Part model, mm, in its own coordinate system. A direction names the side the tool comes from. Round coordinates to 2 decimals unless told otherwise and drop trailing zeros. Order: outer loops, then holes, each group sorted by start corner. A loop starts at its lowest first (then second) coordinate and runs counter-clockwise, first axis right, second up. Notation, with made-up numbers: (-22, 22.5) -> (10, 22.5) arc R15 ccw to (10, 47.5) -> close; hole circle Ø3 at (75, 70). An arc over 180 degrees is marked (long way). Return JSON: item names as keys, results as strings. Group by question number.
from build123d import *

# Parameters (mm, degrees)
SKETCH1_R           = 114.3
BOSS_EXTRUDE1_DEPTH = 76.2
SKETCH2_R           = 88.9
BOSS_EXTRUDE2_DEPTH = 25.4
SKETCH3_W           = 67.503621206
SKETCH3_H           = 186.628871474
BOSS_EXTRUDE3_DEPTH = 203.2
SKETCH4_R           = 76.2
CUT_EXTRUDE1_DEPTH  = 127
FILLET1_SIZE        = 25.4
FILLET2_SIZE        = 12.7


with BuildPart() as part:
    # Sketch1 → Boss-Extrude1 (new body)
    with BuildSketch(Plane(origin=(0, 0, 0), x_dir=(1, 0, 0), z_dir=(0, 1, 0))):
        with Locations(Location((0, 0, 0), (0, 0, 90))):
            Circle(SKETCH1_R)
    extrude(amount=BOSS_EXTRUDE1_DEPTH)

    # Sketch2 → Boss-Extrude2 (add)
    with BuildSketch(Plane(origin=(0, 0, 0), x_dir=(-1, 0, 0), z_dir=(0, -1, 0))):
        with Locations(Location((0, 0, 0), (0, 0, 90))):
            Circle(SKETCH2_R)
    extrude(amount=BOSS_EXTRUDE2_DEPTH)

    # Sketch3 → Boss-Extrude3 (add)
    with BuildSketch(Plane(origin=(0, 76.2, 0), x_dir=(1, 0, 0), z_dir=(0, 1, 0))):
        Rectangle(SKETCH3_W, SKETCH3_H)
    extrude(amount=BOSS_EXTRUDE3_DEPTH)

    # Sketch4 → Cut-Extrude1 (cut)
    with BuildSketch(Plane.ZY.offset(33.751810603)):
        with Locations((0, 177.8)):
            Circle(SKETCH4_R)
    extrude(amount=-CUT_EXTRUDE1_DEPTH, mode=Mode.SUBTRACT)

    # Fillet1
    # a fillet whose section is not a circle: 25.4 mm, written as the material it takes off along each edge
    with BuildSketch(Plane(origin=(97.251810603, 279.4, 93.314435737), x_dir=(0, -1, 0), z_dir=(-1, 0, 0)), Plane(origin=(-97.251810603, 279.4, -93.314435737), x_dir=(0, -1, 0), z_dir=(1, 0, 0))) as fillet1_piece_1:
        with BuildLine():
            Bezier((FILLET1_SIZE, 0), (0, 0), (0, -FILLET1_SIZE), weights=[1, 1, 1])
            Line((0, -FILLET1_SIZE), (0, 0))
            Line((0, 0), (FILLET1_SIZE, 0))
        make_face()
    extrude(amount=194.503621206, mode=Mode.SUBTRACT)

    # Fillet2
    # a fillet whose section is not a circle: 12.7 mm, written as the material it adds along each edge
    with BuildSketch(Plane(origin=(33.751810603, 76.2, 93.314435737), x_dir=(0, 0, 1), z_dir=(-1, 0, 0)), Plane(origin=(-33.751810603, 76.2, -93.314435737), x_dir=(0, 0, -1), z_dir=(1, 0, 0))) as fillet2_piece_1:
        with BuildLine():
            Bezier((FILLET2_SIZE, 0), (0, 0), (0, FILLET2_SIZE), weights=[1, 1, 1])
            Line((0, FILLET2_SIZE), (0, 0))
            Line((0, 0), (FILLET2_SIZE, 0))
        make_face()
    extrude(amount=67.503621206)
    with BuildSketch(Plane(origin=(-33.751810603, 76.2, 93.314435737), x_dir=(-1, 0, 0), z_dir=(0, 0, -1)), Plane(origin=(33.751810603, 76.2, -93.314435737), x_dir=(1, 0, 0), z_dir=(0, 0, 1))) as fillet2_piece_2:
        with BuildLine():
            Bezier((FILLET2_SIZE, 0), (0, 0), (0, FILLET2_SIZE), weights=[1, 1, 1])
            Line((0, FILLET2_SIZE), (0, 0))
            Line((0, 0), (FILLET2_SIZE, 0))
        make_face()
    extrude(amount=186.628871474)
    with BuildSketch(Plane(origin=(65.501810603, 76.2, 93.314435737), x_dir=(0, 0, 1), z_dir=(-1, 0, 0))) as fillet2_piece_3a_section:
        with BuildLine():
            Bezier((FILLET2_SIZE, 0), (0, 0), (0, FILLET2_SIZE), weights=[1, 1, 1])
            Line((0, FILLET2_SIZE), (0, 0))
            Line((0, 0), (FILLET2_SIZE, 0))
        make_face()
    fillet2_piece_3a = extrude(amount=99.253621206, mode=Mode.PRIVATE)
    fillet2_piece_3a = fillet2_piece_3a & Plane(origin=(0, 76.2, 0), x_dir=(0, 0, -1), z_dir=(0, -1, 0)) * Cylinder(114.3, 250, mode=Mode.PRIVATE)
    fillet2_piece_3a = split(fillet2_piece_3a, bisect_by=Plane(origin=(33.751810603, 76.2, 93.314435737), z_dir=(1, 0, 0)), keep=Keep.TOP, mode=Mode.PRIVATE)
    with BuildSketch(Plane(origin=(33.751810603, 76.2, -93.314435737), x_dir=(1, 0, 0), z_dir=(0, 0, 1))) as fillet2_piece_3b_section:
        with BuildLine():
            Bezier((FILLET2_SIZE, 0), (0, 0), (0, FILLET2_SIZE), weights=[1, 1, 1])
            Line((0, FILLET2_SIZE), (0, 0))
            Line((0, 0), (FILLET2_SIZE, 0))
        make_face()
    fillet2_piece_3b = extrude(amount=218.378871474, mode=Mode.PRIVATE)
    fillet2_piece_3b = fillet2_piece_3b & Plane(origin=(0, 76.2, 0), x_dir=(0, 0, -1), z_dir=(0, -1, 0)) * Cylinder(114.3, 488, mode=Mode.PRIVATE)
    fillet2_piece_3b = split(fillet2_piece_3b, bisect_by=Plane(origin=(33.751810603, 76.2, 93.314435737), z_dir=(0, 0, 1)), keep=Keep.TOP, mode=Mode.PRIVATE)
    fillet2_piece_3 = fillet2_piece_3a & fillet2_piece_3b
    add(fillet2_piece_3)
    with BuildSketch(Plane(origin=(-33.751810603, 76.2, 125.064435737), x_dir=(-1, 0, 0), z_dir=(0, 0, -1))) as fillet2_piece_4a_section:
        with BuildLine():
            Bezier((FILLET2_SIZE, 0), (0, 0), (0, FILLET2_SIZE), weights=[1, 1, 1])
            Line((0, FILLET2_SIZE), (0, 0))
            Line((0, 0), (FILLET2_SIZE, 0))
        make_face()
    fillet2_piece_4a = extrude(amount=218.378871474, mode=Mode.PRIVATE)
    fillet2_piece_4a = fillet2_piece_4a & Plane(origin=(0, 76.2, 0), x_dir=(0, 0, -1), z_dir=(0, -1, 0)) * Cylinder(114.3, 488, mode=Mode.PRIVATE)
    fillet2_piece_4a = split(fillet2_piece_4a, bisect_by=Plane(origin=(-33.751810603, 76.2, 93.314435737), z_dir=(0, 0, 1)), keep=Keep.TOP, mode=Mode.PRIVATE)
    with BuildSketch(Plane(origin=(33.751810603, 76.2, 93.314435737), x_dir=(0, 0, 1), z_dir=(-1, 0, 0))) as fillet2_piece_4b_section:
        with BuildLine():
            Bezier((FILLET2_SIZE, 0), (0, 0), (0, FILLET2_SIZE), weights=[1, 1, 1])
            Line((0, FILLET2_SIZE), (0, 0))
            Line((0, 0), (FILLET2_SIZE, 0))
        make_face()
    fillet2_piece_4b = extrude(amount=99.253621206, mode=Mode.PRIVATE)
    fillet2_piece_4b = fillet2_piece_4b & Plane(origin=(0, 76.2, 0), x_dir=(0, 0, -1), z_dir=(0, -1, 0)) * Cylinder(114.3, 250, mode=Mode.PRIVATE)
    fillet2_piece_4b = split(fillet2_piece_4b, bisect_by=Plane(origin=(-33.751810603, 76.2, 93.314435737), z_dir=(-1, 0, 0)), keep=Keep.TOP, mode=Mode.PRIVATE)
    fillet2_piece_4 = fillet2_piece_4a & fillet2_piece_4b
    add(fillet2_piece_4)
    with BuildSketch(Plane(origin=(-33.751810603, 76.2, 93.314435737), x_dir=(-1, 0, 0), z_dir=(0, 0, -1))) as fillet2_piece_5a_section:
        with BuildLine():
            Bezier((FILLET2_SIZE, 0), (0, 0), (0, FILLET2_SIZE), weights=[1, 1, 1])
            Line((0, FILLET2_SIZE), (0, 0))
            Line((0, 0), (FILLET2_SIZE, 0))
        make_face()
    fillet2_piece_5a = extrude(amount=218.378871474, mode=Mode.PRIVATE)
    fillet2_piece_5a = fillet2_piece_5a & Plane(origin=(0, 76.2, 0), x_dir=(0, 0, -1), z_dir=(0, -1, 0)) * Cylinder(114.3, 488, mode=Mode.PRIVATE)
    fillet2_piece_5a = split(fillet2_piece_5a, bisect_by=Plane(origin=(-33.751810603, 76.2, -93.314435737), z_dir=(0, 0, -1)), keep=Keep.TOP, mode=Mode.PRIVATE)
    with BuildSketch(Plane(origin=(-65.501810603, 76.2, -93.314435737), x_dir=(0, 0, -1), z_dir=(1, 0, 0))) as fillet2_piece_5b_section:
        with BuildLine():
            Bezier((FILLET2_SIZE, 0), (0, 0), (0, FILLET2_SIZE), weights=[1, 1, 1])
            Line((0, FILLET2_SIZE), (0, 0))
            Line((0, 0), (FILLET2_SIZE, 0))
        make_face()
    fillet2_piece_5b = extrude(amount=99.253621206, mode=Mode.PRIVATE)
    fillet2_piece_5b = fillet2_piece_5b & Plane(origin=(0, 76.2, 0), x_dir=(0, 0, -1), z_dir=(0, -1, 0)) * Cylinder(114.3, 250, mode=Mode.PRIVATE)
    fillet2_piece_5b = split(fillet2_piece_5b, bisect_by=Plane(origin=(-33.751810603, 76.2, -93.314435737), z_dir=(-1, 0, 0)), keep=Keep.TOP, mode=Mode.PRIVATE)
    fillet2_piece_5 = fillet2_piece_5a & fillet2_piece_5b
    add(fillet2_piece_5)
    with BuildSketch(Plane(origin=(33.751810603, 76.2, -125.064435737), x_dir=(1, 0, 0), z_dir=(0, 0, 1))) as fillet2_piece_6a_section:
        with BuildLine():
            Bezier((FILLET2_SIZE, 0), (0, 0), (0, FILLET2_SIZE), weights=[1, 1, 1])
            Line((0, FILLET2_SIZE), (0, 0))
            Line((0, 0), (FILLET2_SIZE, 0))
        make_face()
    fillet2_piece_6a = extrude(amount=218.378871474, mode=Mode.PRIVATE)
    fillet2_piece_6a = fillet2_piece_6a & Plane(origin=(0, 76.2, 0), x_dir=(0, 0, -1), z_dir=(0, -1, 0)) * Cylinder(114.3, 488, mode=Mode.PRIVATE)
    fillet2_piece_6a = split(fillet2_piece_6a, bisect_by=Plane(origin=(33.751810603, 76.2, -93.314435737), z_dir=(0, 0, -1)), keep=Keep.TOP, mode=Mode.PRIVATE)
    with BuildSketch(Plane(origin=(-33.751810603, 76.2, -93.314435737), x_dir=(0, 0, -1), z_dir=(1, 0, 0))) as fillet2_piece_6b_section:
        with BuildLine():
            Bezier((FILLET2_SIZE, 0), (0, 0), (0, FILLET2_SIZE), weights=[1, 1, 1])
            Line((0, FILLET2_SIZE), (0, 0))
            Line((0, 0), (FILLET2_SIZE, 0))
        make_face()
    fillet2_piece_6b = extrude(amount=99.253621206, mode=Mode.PRIVATE)
    fillet2_piece_6b = fillet2_piece_6b & Plane(origin=(0, 76.2, 0), x_dir=(0, 0, -1), z_dir=(0, -1, 0)) * Cylinder(114.3, 250, mode=Mode.PRIVATE)
    fillet2_piece_6b = split(fillet2_piece_6b, bisect_by=Plane(origin=(33.751810603, 76.2, -93.314435737), z_dir=(1, 0, 0)), keep=Keep.TOP, mode=Mode.PRIVATE)
    fillet2_piece_6 = fillet2_piece_6a & fillet2_piece_6b
    add(fillet2_piece_6)


solid = part.part
(1) Tool access for faces 4 (the flat face through (-73, 76.2, 1)), 5 (the flat face through (72, 76.2, 1)), 6 (the flat face through (0, 170, -93.314)), 7 (the flat face through (67, 0, -59)): list every direction of +Z, -Z, +X, -X, +Y, -Y with a clear straight run to the whole face (end or side of a thin tool).
(2) Saw through at C-C, the plane y = 6.5. List the corners of the cut face in (x, z), and give its area (3 significant figures).
(3) Saw through at D-D, the plane x = 77. List the corners of the cut face in (y, z).
(4) Mould opens along Z. For faces 1 (the cylindrical face through (-0.47, 253.35, -9.92)), 2 (the cylindrical face through (74.96, -12.52, -47.79)), 3 (the flat face through (33.752, 249, -43)) say: pulls with the +Z half, pulls with the -Z half, needs draft (parallel to the pull), parting line crosses it, or undercut.
(5) Probe L1, parallel to Z at x = 12, y = 177; L2, parallel to Y at x = 0, z = 0; L3, parallel to Y at x = 96.5, z = -13.5. List the from-to ranges inside material, lowest first. Write a range as [from, to].
(6) Pin check, flat tips, straight feed: P1, Ø5, axis at x = -27.5, y = 224.5, coming from the -Z side; P2, Ø9, axis at x = -12.5, z = 110, coming from the +Y side; P3, Ø10, axis at x = -71.5, z = 66, coming from the -Y side. Stop position of each tip, or through.
(7) Saw through at A-A, the plane y = 177.8. List the corners of the cut face in (x, z).
(8) Saw through at B-B, the plane x = -63. List the corners of the cut face in (y, z), and give its area (3 significant figures).
Results are:
{
 "1": {"face 4": "+Z, -Z, -X, +Y", "face 5": "+Z, -Z, +X, +Y", "face 6": "-Z, +X, -X, +Y", "face 7": "-Y"},
 "2": {"outline": "circle Ø228.6 at (0, 0)", "area": "41,000 mm^2"},
 "3": {"outline": "(-25.4, -44.43) -> (0, -44.43) -> (0, -84.47) -> (76.2, -84.47) -> (76.2, 84.47) -> (0, 84.47) -> (0, 44.43) -> (-25.4, 44.43) -> close"},
 "4": {"face 1": "undercut", "face 2": "parting line crosses it", "face 3": "needs draft"},
 "5": {"L1": "z = [-93.31, -76.2], [76.2, 93.31]", "L2": "y = [-25.4, 101.6], [254, 279.4]", "L3": "y = [0, 76.2]"},
 "6": {"P1": "stops at z = -93.31", "P2": "stops at y = 76.21", "P3": "stops at y = 0"},
 "7": {"outline": "(-33.75, -93.31) -> (33.75, -93.31) -> (33.75, -76.2) -> (-33.75, -76.2) -> close; (-33.75, 76.2) -> (33.75, 76.2) -> (33.75, 93.31) -> (-33.75, 93.31) -> close"},
 "8": {"outline": "(-25.4, -62.72) -> (0, -62.72) -> (0, -95.37) -> (76.2, -95.37) -> (76.2, 95.37) -> (0, 95.37) -> (0, 62.72) -> (-25.4, 62.72) -> close", "area": "17,700 mm^2"}
}
